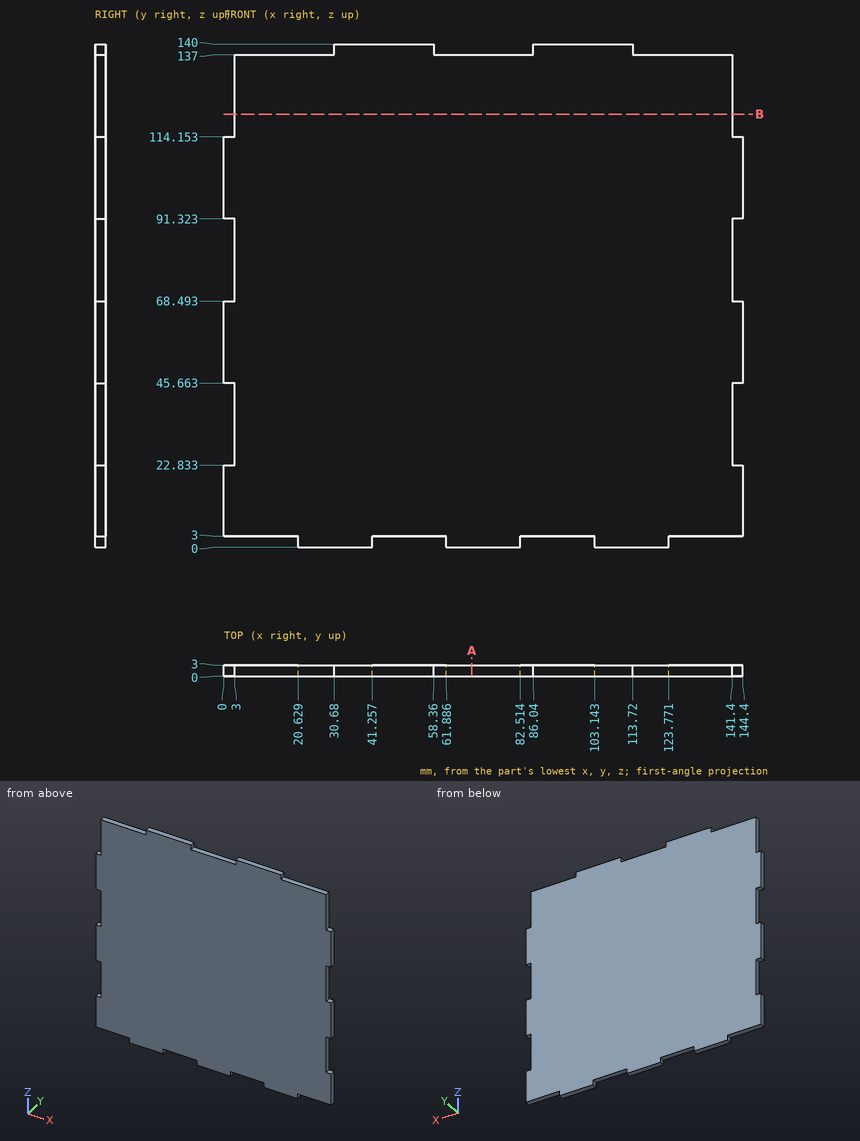
Here's the drawing with two shaded views (mm, measured from the low corner). I have some questions. Coordinates: 2 decimals unless noted, no trailing zeros. Order: outer loops, then holes, each group sorted by start corner. A loop starts at its lowest first (then second) coordinate and runs counter-clockwise, first axis right, second up.
Item 1: If we section it at A-A on x = 69: List the corners of the cut face in (y, z) for me.
Result sheet:
outline: (0, 0) - (3, 0) - (3, 137) - (0, 137) - close
Item 2: If we section it at B-B on z = 120.5: List the corners of the cut face in (x, y) for me.
Result sheet:
outline: (3, 0) - (141.4, 0) - (141.4, 3) - (3, 3) - close
Item 3: For P1, Ø1.5, axis at x = 53, y = 2, coming from the -Z side; P2, Ø10, axis at x = 93.5, z = 122, coming from the -Y side; P3, Ø1.5, axis at x = 2, y = 1, coming from the +Z side; P4, Ø1.5, axis at x = 123.5, y = 2, coming from the +Z side, each with a flat end and sliding along its axis, tell me the tip position at first contact or that it passes through.
Result sheet:
P1: stops at z = 3
P2: stops at y = 0
P3: stops at z = 114.15
P4: stops at z = 137
Item 4: I need wall thicknesses on line 1 (Z direction, x = 21.5, y = 1); line 2 (X direction, y = 1, z = 89); line 3 (Z direction, x = 124, y = 0.6). Which ranges of each line are inside material? Lowest first, please.
Result sheet:
line 1: z = 0 to 137
line 2: x = 3 to 141.4
line 3: z = 3 to 137
